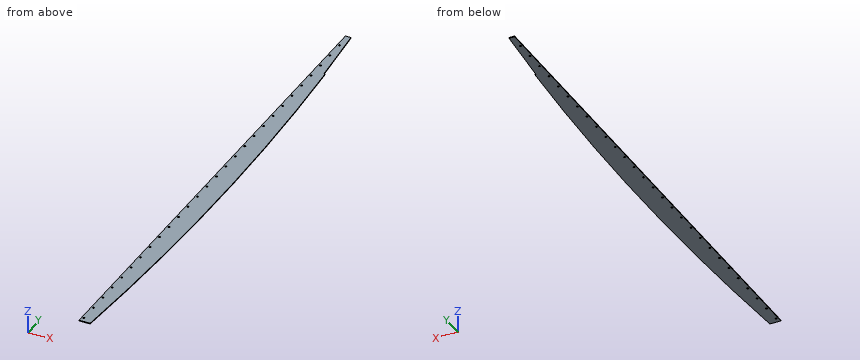
Autodesk Inventor part; units mm, degrees
ref_plane "YZ Plane" through (0, 0, 0) normal (1, 0, 0) x (0, 1, 0)
ref_plane "XZ Plane" through (0, 0, 0) normal (0, 1, 0) x (-1, 0, 0)
ref_plane "XY Plane" through (0, 0, 0) normal (0, 0, 1) x (1, 0, 0)
sketch "Sketch1" plane through (0, 0, 0) normal (0, 0, 1) x (1, 0, 0)
  line L0 (0, 100) -> (0, 50) construction
  line L1 (0, 47) -> (0, 0) construction
  line L2 (0, 50) -> (0, 47) construction
  arc A0 (42, -1970) -> (25, 0) centre (-10972.0978, -1079.9722) ccw
  line L3 (42, -1970) -> (0, -1970)
  line L4 (0, -1970) -> (0, 0)
  line L5 (0, 0) -> (25, 0)
  line L6 (21, 0) -> (41.9305, -240)
  line L7 (41.9305, -240) -> (45.9305, -240)
  dimension "d115" = 3
  dimension "d131" = 11050
  dimension "d132" = 25
  dimension "d133" = 42
  dimension "d134" = 1970
  dimension "d145" = 4
  dimension "d146" = 240
  dimension "d147" = 4
extrude "Plate3" add sketch "Sketch1" along normal blind 3 contours L3 L4 L5 L6 L7 A0
sketch "Sketch3" plane through (0, 0, 0) normal (0, 0, -1) x (-1, 0, 0)
  line L0 (0, 0) -> (0, -1970)
  line L1 (-21, 0) -> (0, 0)
  arc A0 (-45.9305, -240) -> (-42, -1970) centre (10972.0978, -1079.9722) ccw
  line L2 (0, -1970) -> (-42, -1970)
  circle A1 centre (-8, -1950) radius 3.5
  circle A2 centre (0, -1947.1277) radius 5
  circle A3 centre (0, -1947.1277) radius 12
  line L3 (-41.9305, -240) -> (-21, 0)
  line L4 (-45.9305, -240) -> (-41.9305, -240)
  point P0 (0, -1935.1277)
  point P1 (-11.2941, -1951.1827)
  point P2 (-4.7059, -1948.8173)
  point P3 (0, -1942.1277)
  dimension "d135" = 7
  dimension "d136" = 8
  dimension "d137" = 20
  dimension "d143" = 10
extrude "Extrusion2" cut sketch "Sketch3" against normal blind 10 contours A1
pattern_linear "Rectangular Pattern1" count 31 spacing 70 along (0, 1, 0) of "Extrusion2"
equation "\"BendReliefWidth\" = Thickness"
equation "\"BendReliefDepth\" = 0.5 * Thickness"
equation "\"CornerReliefSize\" = 4 * Thickness"
equation "\"MinimumRemnant\" = 2 * Thickness"
equation "\"GapSize\" = Thickness"
properties part number "MSC 813 WALL SUPPORT GILLS" material "AISI304"
Source: CAD feature listing. Evaluate the final solid. Frame: model axes, mm. Give positions to 0.01 mm unless a question says otherwise; leave off trailing zeros. Order: outer loops, then holes, each group sorted by start corner. A loop starts at its lowest first (then second) coordinate and runs counter-clockwise, first axis right, second up. Notation, with made-up numbers: (-6.75, 0.5) -> (2.25, 0.5) arc R33 ccw to (2.25, 34.5) -> close; hole circle Ø4 at (82, -27.75). An arc over 180 degrees is marked (long way). Write item = value, one per line.
Q1. Cut plane A-A, the plane z = 1.95. State how many separate pieces and enclosed holes the cut face has, and give its area (3 significant figures).
Data:
separate_pieces = 1
enclosed_holes = 28
area = 122,000 mm^2
Q2. Pin query (flat end, axial travel): pin 1 (6.5 mm diameter, centred on x = 8, y = -1110, fed in from -Z). Return the tip coordinate at first contact, or that it passes through.
Data:
pin_1 = through
Q3. Cut plane B-B, the plane y = -1436. Output: boundary loops of the cut face in (x, z).
Data:
outline = (0, 0) -> (72.17, 0) -> (72.17, 3) -> (0, 3) -> close
Q4. Material intervals for line 1 (X direction, y = -1014, z = 0.95); line 2 (X direction, y = -1040, z = 1); line 3 (X direction, y = -970, z = 1.9), sorted ascending. Write a range as from..to.
Data:
line_1 = 0..77.71
line_2 = 0..4.5, 11.5..77.83
line_3 = 0..4.5, 11.5..77.35
